```python
from build123d import *

# Parameters (mm, degrees)
SKETCH_1_R          = 5
SKETCH_1_R_2        = 2.5
EXTRUDE_1_DEPTH     = 9
SKETCH_2_R          = 3.75
CUT_EXTRUDE_1_DEPTH = 2
SKETCH_3_R          = 2.9
EXTRUDE_2_DEPTH     = 3
FILLET_1_R          = 2
SKETCH_4_R          = 2.9
EXTRUDE_3_DEPTH     = 5
FILLET_2_R          = 2.9


with BuildPart() as part:
    # 스케치1 → 보스-돌출1 (new body)
    # profile 1 of 5: a face of its own
    with BuildSketch(Plane.XY):
        with BuildLine():
            Line((8.866410343, 21.94338903), (4.384187039, 21.94338903))
            Line((4.384187039, 21.94338903), (2.987768149, 19.65002342))
            Line((2.987768149, 19.65002342), (2.987768149, 17.661246793))
            Line((2.987768149, 17.661246793), (2.987768149, 9.70876495))
            Line((2.987768149, 9.70876495), (-3.184671245, 3.854590647))
            ThreePointArc((-3.184671245, 3.854590647), (2.13033375, 4.523458645), (5, 0))
            ThreePointArc((5, 0), (0, -5), (-5, 0))
            Line((-5, 0), (-5, -14.85442617))
            Line((-5, -14.85442617), (-19.921487255, -13.496967469))
            ThreePointArc((-19.921487255, -13.496967469), (-21.453925628, -14.014242075), (-22.102673306, -15.49581787))
            ThreePointArc((-22.102673306, -15.49581787), (-21.54079944, -16.765444299), (-20.287735083, -17.363343312))
            Line((-20.287735083, -17.363343312), (-13.716958703, -17.9611093))
            ThreePointArc((-13.716958703, -17.9611093), (-10.295562947, -19.77999502), (-9.201017746, -23.497018692))
            Line((-9.201017746, -23.497018692), (-8.648726299, -43.504972105))
            ThreePointArc((-8.648726299, -43.504972105), (-4.194233385, -55.315987694), (5.178631732, -63.771281648))
            ThreePointArc((5.178631732, -63.771281648), (9.354068035, -62.453221011), (8.453005262, -58.168406191))
            ThreePointArc((8.453005262, -58.168406191), (-0.467627925, -43.39335713), (3.924251711, -26.702306699))
            Line((3.924251711, -26.702306699), (8.3701186, -14.978169718))
            ThreePointArc((8.3701186, -14.978169718), (8.662275884, -14.729272874), (8.69193724, -14.346616734))
            ThreePointArc((8.69193724, -14.346616734), (8.365752146, -12.021808556), (8.866410343, -9.728236855))
            Line((8.866410343, -9.728236855), (8.866410343, 21.94338903))
        make_face()
    # profile 2 of 5: a face of its own
    with BuildSketch(Plane.XY):
        Circle(SKETCH_1_R)
        Circle(SKETCH_1_R_2, mode=Mode.SUBTRACT)
    # profile 3 of 5: a face of its own
    with BuildSketch(Plane.XY):
        with BuildLine():
            ThreePointArc((5, 0), (2.13033375, 4.523458645), (-3.184671245, 3.854590647))
            ThreePointArc((-3.184671245, 3.854590647), (-4.523458645, 2.13033375), (-5, 0))
            ThreePointArc((-5, 0), (0, -5), (5, 0))
        make_face()
        Circle(SKETCH_1_R_2, mode=Mode.SUBTRACT)
    # profile 4 of 5: a face of its own
    with BuildSketch(Plane.XY):
        Polygon((8.866410343, 24.501339074), (6.942137083, 24.501339074), (4.384187039, 21.94338903), (8.866410343, 21.94338903), align=None)
    # profile 5 of 5: a face of its own
    with BuildSketch(Plane.XY):
        with BuildLine():
            Line((8.866410343, 21.94338903), (4.384187039, 21.94338903))
            Line((4.384187039, 21.94338903), (2.987768149, 19.65002342))
            Line((2.987768149, 19.65002342), (2.987768149, 17.661246793))
            Line((2.987768149, 17.661246793), (2.987768149, 9.70876495))
            Line((2.987768149, 9.70876495), (-3.184671245, 3.854590647))
            ThreePointArc((-3.184671245, 3.854590647), (2.13033375, 4.523458645), (5, 0))
            ThreePointArc((5, 0), (0, -5), (-5, 0))
            Line((-5, 0), (-5, -14.85442617))
            Line((-5, -14.85442617), (-19.921487255, -13.496967469))
            ThreePointArc((-19.921487255, -13.496967469), (-21.453925628, -14.014242075), (-22.102673306, -15.49581787))
            ThreePointArc((-22.102673306, -15.49581787), (-21.54079944, -16.765444299), (-20.287735083, -17.363343312))
            Line((-20.287735083, -17.363343312), (-13.716958703, -17.9611093))
            ThreePointArc((-13.716958703, -17.9611093), (-10.295562947, -19.77999502), (-9.201017746, -23.497018692))
            Line((-9.201017746, -23.497018692), (-8.648726299, -43.504972105))
            ThreePointArc((-8.648726299, -43.504972105), (-4.194233385, -55.315987694), (5.178631732, -63.771281648))
            ThreePointArc((5.178631732, -63.771281648), (9.354068035, -62.453221011), (8.453005262, -58.168406191))
            ThreePointArc((8.453005262, -58.168406191), (-0.467627925, -43.39335713), (3.924251711, -26.702306699))
            Line((3.924251711, -26.702306699), (8.3701186, -14.978169718))
            ThreePointArc((8.3701186, -14.978169718), (8.662275884, -14.729272874), (8.69193724, -14.346616734))
            ThreePointArc((8.69193724, -14.346616734), (8.365752146, -12.021808556), (8.866410343, -9.728236855))
            Line((8.866410343, -9.728236855), (8.866410343, 21.94338903))
        make_face()
    extrude(amount=EXTRUDE_1_DEPTH)

    # 스케치2 → 컷-돌출1 (cut)
    with BuildSketch(Plane(origin=(8.866410343, 0, 0), x_dir=(0, 0, -1), z_dir=(1, 0, 0))):
        with Locations(Location((-4.5, 14.501339074, 0), (0, 0, 90))):
            Circle(SKETCH_2_R)
    extrude(amount=-CUT_EXTRUDE_1_DEPTH, mode=Mode.SUBTRACT)

    # 스케치3 → 보스-돌출2 (add)
    with BuildSketch(Plane(origin=(6.866410343, 0, 0), x_dir=(0, 0, -1), z_dir=(1, 0, 0))):
        with Locations(Location((-4.5, 14.501339074, 0), (0, 0, 90))):
            Circle(SKETCH_3_R)
    extrude(amount=EXTRUDE_2_DEPTH)

    # 필렛1
    fillet_1_edges = [part.edges().sort_by_distance(p)[0] for p in [
        (9.866410343, 11.601339074, 4.5),
    ]]
    fillet(fillet_1_edges, radius=FILLET_1_R)

    # 스케치4 → 보스-돌출3 (add)
    with BuildSketch(Plane(origin=(-1.381306819, -15.183631058, 0), x_dir=(0.995887428286197, -0.09059928355955607, 0), z_dir=(0.09059928355955607, 0.995887428286197, 0))):
        with Locations((-10.133636773, -4.5)):
            Circle(SKETCH_4_R)
    extrude(amount=EXTRUDE_3_DEPTH)

    # 필렛2
    fillet_2_edges = [part.edges().sort_by_distance(p)[0] for p in [
        (-13.908345408, -9.023355763, 4.5),
    ]]
    fillet(fillet_2_edges, radius=FILLET_2_R)


solid = part.part
```
The model under review builds one solid part; all positions refer to its coordinate system, in mm. A direction names the side the tool comes from. Round coordinates to 2 decimals unless told otherwise and drop trailing zeros. Order: outer loops, then holes, each group sorted by start corner. A loop starts at its lowest first (then second) coordinate and runs counter-clockwise, first axis right, second up. Notation, with made-up numbers: (7.5, 59.5) - (47.5, 59.5) arc R28 cw to (47.5, 89.5) - close; hole circle Ø8 at (77, 22). An arc over 180 degrees is marked (long way). Answer in a Markdown table with one row per item.
(1) Clearance check with flat-ended pins moving along their axes: P1, Ø3, axis at x = -16.5, z = 4, coming from the +Y side; P2, Ø1, axis at y = -36, z = 3.5, coming from the -X side; P3, Ø2.5, axis at y = 4.5, z = 3.5, coming from the +X side. State where each tip first meets the part, or that it passes through.
Result set:
| item | result |
|---|---|
| P1 | stops at y = -13.67 |
| P2 | stops at x = -8.87 |
| P3 | stops at x = 8.87 |
(2) Take a section at B-B on x = -17. Write out the cut boundary in (y, z), plus the area to 3 significant figures.
Result set:
| item | result |
|---|---|
| outline | (-17.66, 0) - (-13.76, 0) - (-13.76, 9) - (-17.66, 9) - close |
| area | 35.1 mm2 |
(3) Mouldability with a two-part tool opening along Y and no side actions: class faces 1 (the face through (8, 24.501, 4)), 2 (the face through (2.988, 15, 4)), 3 (the face through (8.866, 7, 4)) as released by +Y, released by -Y, zero draft, split by the parting line, or undercut.
Result set:
| item | result |
|---|---|
| face 1 | released by +Y |
| face 2 | zero draft |
| face 3 | undercut |
(4) Machinability: for faces 4 (the face through (6.116, -20.922, 4.437)), 5 (the face through (9.866, 14, 5)), 6 (the face through (7.359, 17.267, 5.371)), 7 (the face through (5.68, 23.24, 4.44)), 8 (the face through (-5, -7, 4)), which of the approach directions +Z, -Z, +X, -X, +Y, -Y give a long, thin tool a straight path to every point of the face, cutting with its end or side? Answer none if there is none.
Result set:
| item | result |
|---|---|
| face 4 | +Z, -Z, +X |
| face 5 | +Z, -Z, +X, +Y, -Y |
| face 6 | +X |
| face 7 | +Z, -Z, -X, +Y |
| face 8 | +Z, -Z, +Y |
(5) For line 1 (Y direction, x = 1, z = 7.75); line 2 (X direction, y = -7, z = 5.5); line 3 (X direction, y = 12, z = 0.75), list the stretches that pass through material, from the lowest coordinate up. Write a range as from..to.
Result set:
| item | result |
|---|---|
| line 1 | y = -60.97..-48.73, -31.74..-2.29, 2.29..7.82 |
| line 2 | x = -5..8.87 |
| line 3 | x = 2.99..8.87 |
(6) Take a section at A-A on y = -40. Write out the cut boundary in (x, z).
Result set:
| item | result |
|---|---|
| outline | (-8.75, 0) - (-0.69, 0) - (-0.69, 9) - (-8.75, 9) - close |
